The figure shows three views and two pictorial views of one solid part (mm, origin at its lowest corner). Answer the questions. A direction names the side the tool comes from. Coordinates: 2 decimals unless noted, no trailing zeros. Write each loop counter-clockwise with the first axis right and the second up, starting at its lowest first coordinate (ties: lowest second). Pieces come first, ordered by that corner, then holes.
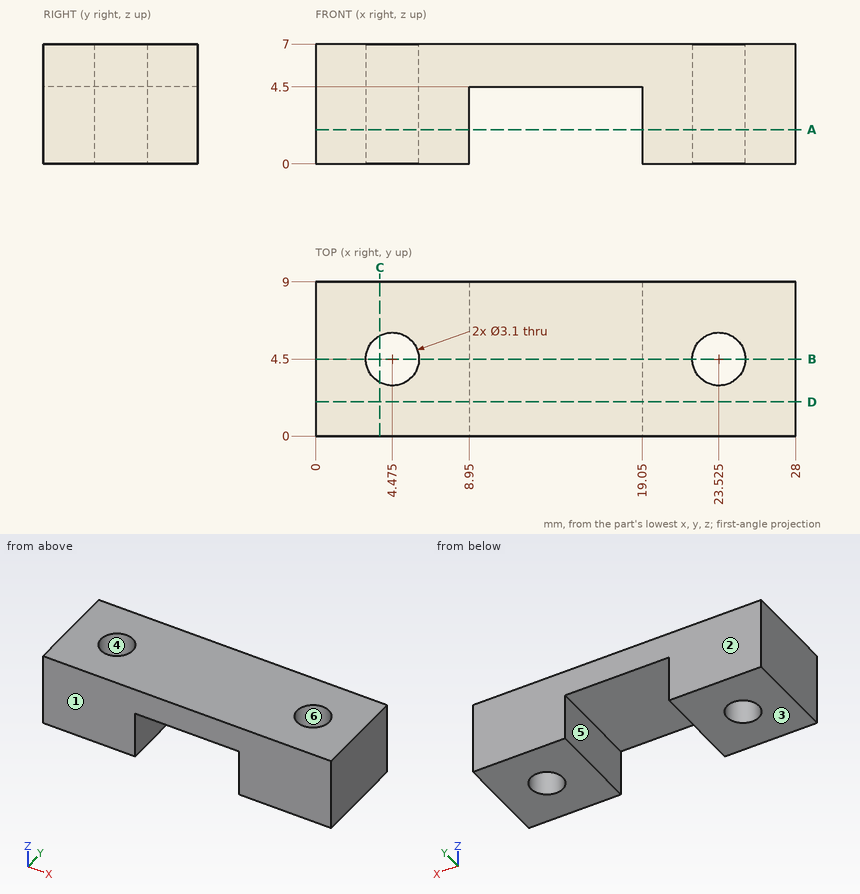
1. Section A-A on z = 2 is taken. Give the vertices of the cut face in (x, y) (3 decimals), then the cut area to 3 significant figures.
Results found:
outline: (0, 0) - (8.95, 0) - (8.95, 9) - (0, 9) - close; (19.05, 0) - (28, 0) - (28, 9) - (19.05, 9) - close; hole circle Ø3.1 at (4.475, 4.5); hole circle Ø3.1 at (23.525, 4.5)
area: 146 mm2
2. A flat-ended cylindrical pin translates along its axis: P1, Ø2.5, axis at x = 12.5, y = 3.5, coming from the -Z side. Find the tip coordinate at first contact, or state that the pin passes through.
Results found:
P1: stops at z = 4.5
3. For a pull along Y with two mould halves and no side action, classify the marked faces 1, 2, 3 and 4 as pulls with the +Y half, pulls with the -Y half, needs draft (parallel to the pull), parting line crosses it, or undercut.
Results found:
face 1: pulls with the -Y half
face 2: pulls with the +Y half
face 3: needs draft
face 4: undercut
4. Section B-B on y = 4.5 is taken. Give the vertices of the cut face in (x, z) (3 decimals), then the cut area to 3 significant figures.
Results found:
outline: (0, 0) - (2.925, 0) - (2.925, 7) - (0, 7) - close; (6.025, 0) - (8.95, 0) - (8.95, 4.5) - (19.05, 4.5) - (19.05, 0) - (21.975, 0) - (21.975, 7) - (6.025, 7) - close; (25.075, 0) - (28, 0) - (28, 7) - (25.075, 7) - close
area: 107 mm2
5. Section C-C on x = 3.75 is taken. Give the vertices of the cut face in (y, z).
Results found:
outline: (0, 0) - (3.13, 0) - (3.13, 7) - (0, 7) - close; (5.87, 0) - (9, 0) - (9, 7) - (5.87, 7) - close
6. A tool of negligible diameter and unlimited length cuts with its end or side. For the marked faces 5 and 6, from which of +Z, -Z, +X, -X, +Y, -Y can it reach the whole face along a straight path? Write none if from no direction.
Results found:
face 5: -Z, +Y, -Y
face 6: +Z, -Z
7. Section D-D on y = 2 is taken. Give the vertices of the cut face in (x, z), then the cut area to 3 significant figures.
Results found:
outline: (0, 0) - (8.95, 0) - (8.95, 4.5) - (19.05, 4.5) - (19.05, 0) - (28, 0) - (28, 7) - (0, 7) - close
area: 151 mm2
8. Find the intervals of material crossed by L1, parallel to X at y = 4.5, z = 3.25 (3 decimals); L2, parallel to X at y = 1.75, z = 2.5; L3, parallel to X at y = 3.25, z = 3, in increasing order.
Results found:
L1: x = 0 to 2.925, 6.025 to 8.95, 19.05 to 21.975, 25.075 to 28
L2: x = 0 to 8.95, 19.05 to 28
L3: x = 0 to 3.56, 5.39 to 8.95, 19.05 to 22.61, 24.44 to 28
